Geometry check sheet. Reference: the model listing, model coordinates, mm. A direction names the side the tool comes from. Round coordinates to 2 decimals unless told otherwise and drop trailing zeros. Loops run counter-clockwise (first coordinate to the right, second up) from the corner with the lowest first, then second, coordinate; pieces in that order, holes last. Notation, with made-up numbers: (68.5, 46.25) - (81.5, 46.25) arc R24 cw to (81.5, 77.25) - close; hole circle Ø9 at (-38.75, 20). An arc over 180 degrees is marked (long way). Answer as CSV lines item,"result". Start each with the question number.
1) Cross-section at D-D on y = -22.25. Record the boundary of the cut face in (x, z).
2) Draft check along X on faces 4 (the flat face through (12.565, -13, 19)), 5 (the flat face through (-7, -25.4, 9)), 6 (the cylindrical face through (-44.58, -12.42, 6.44)). Enter one of: released by +X, released by -X, zero draft, split by the parting line, or undercut.
3) Cross-section at A-A on z = 8.5. Record the boundary of the cut face in (x, y).
4) Cross-section at B-B on y = -15.5. Record the boundary of the cut face in (x, z), and give its area (3 significant figures).
5) Cross-section at C-C on z = 28.5. Record the boundary of the cut face in (x, y), and give its area (3 significant figures).
6) Access from +Z, -Z, +X, -X, +Y, -Y to the whole of each face (thin tool, end or side, straight path). Record for faces 1 (the flat face through (17, -13, 12.7)), 2 (the cylindrical face through (20.226, -16.564, 6.439)), 3 (the flat face through (-32, -15, 12.7)).
7) Depth check by flat-ended pin: P1, Ø5, axis at x = -22.5, z = 29.5, coming from the +Y side; P2, Ø10, axis at x = -38.5, y = -5, coming from the +Z side; P3, Ø7.5, axis at x = 25.27, y = -12.7, coming from the -Z side; P4, Ø8, axis at y = -20.5, z = 6.5, coming from the +X side. Enter the tip coordinate at first touch or a pass-through.
8) Thickness scan on line 1 along Y through (x, z) = (-38.5, 10); line 2 along Z through (x, y) = (32.5, -21.5); line 3 along Y through (x, z) = (-33, 11). Record the ranges inside material, lowest first.
from build123d import *

# Parameters (mm, degrees)
F1_DEPTH  = 25.4
F3_DEPTH  = 25.4
F5_DEPTH  = 25.4
F6_R      = 6.35
F7_DEPTH  = 25.4
F8_R      = 6.35
F9_DEPTH  = 25.4
F10_R     = 6.35
F11_DEPTH = 38.1
F13_DEPTH = 38.1


with BuildPart() as f1:
    # F0 (on Front) → F1 (new body)
    with BuildSketch(Plane.XZ):
        Polygon((-50.9347495013, 12.7), (-50.9347495013, 0), (37.9652504987, 0), (37.9652504987, 12.7), (12.5652504987, 12.7), (12.5652504987, 36.2809036063), (-25.5347495013, 36.2809036063), (-25.5347495013, 12.7), align=None)
    extrude(amount=F1_DEPTH)

    # F2 (on face) → F3 (cut)
    with BuildSketch(Plane.XY.offset(12.7)):
        with BuildLine():
            ThreePointArc((-50.9347495013, -12.7), (-47.2150056224, -3.7197438789), (-38.2347495013, 0))
            Line((-38.2347495013, 0), (-50.9347495013, 0))
            Line((-50.9347495013, 0), (-50.9347495013, -12.7))
        make_face()
        with BuildLine():
            Line((-50.9347495013, -25.4), (-38.2347495013, -25.4))
            ThreePointArc((-38.2347495013, -25.4), (-47.2150056224, -21.6802561211), (-50.9347495013, -12.7))
            Line((-50.9347495013, -12.7), (-50.9347495013, -25.4))
        make_face()
    extrude(amount=-F3_DEPTH, mode=Mode.SUBTRACT)

    # F4 (on face) → F5 (cut)
    with BuildSketch(Plane.XY.offset(12.7)):
        with BuildLine():
            ThreePointArc((25.2652504987, 0), (34.2455066198, -3.7197438789), (37.9652504987, -12.7))
            Line((37.9652504987, -12.7), (37.9652504987, 0))
            Line((37.9652504987, 0), (25.2652504987, 0))
        make_face()
        with BuildLine():
            Line((37.9652504987, -25.4), (37.9652504987, -12.7))
            ThreePointArc((37.9652504987, -12.7), (34.2455066198, -21.6802561211), (25.2652504987, -25.4))
            Line((25.2652504987, -25.4), (37.9652504987, -25.4))
        make_face()
    extrude(amount=-F5_DEPTH, mode=Mode.SUBTRACT)

    # F6 (on face) → F7 (cut)
    with BuildSketch(Plane.XY.offset(12.7)):
        with Locations((-38.2347495013, -12.7)):
            Circle(F6_R)
    extrude(amount=-F7_DEPTH, mode=Mode.SUBTRACT)

    # F8 (on face) → F9 (cut)
    with BuildSketch(Plane.XY.offset(12.7)):
        with Locations((25.2652504987, -12.7)):
            Circle(F8_R)
    extrude(amount=-F9_DEPTH, mode=Mode.SUBTRACT)

    # F10 (on face) → F11 (cut)
    with BuildSketch(Plane.YZ.offset(12.5652504987)):
        with Locations((-12.7911586314, 26.1209036063)):
            Circle(F10_R)
    extrude(amount=-F11_DEPTH, mode=Mode.SUBTRACT)

    # F12 (on face) → F13 (cut)
    with BuildSketch(Plane.YZ.offset(12.5652504987)):
        with BuildLine():
            ThreePointArc((-25.4, 23.5809036063), (-21.6802561211, 32.5611597274), (-12.7, 36.2809036063))
            Line((-12.7, 36.2809036063), (-25.4, 36.2809036063))
            Line((-25.4, 36.2809036063), (-25.4, 23.5809036063))
        make_face()
        with BuildLine():
            ThreePointArc((-12.7, 36.2809036063), (-3.7197438789, 32.5611597274), (0, 23.5809036063))
            Line((0, 23.5809036063), (0, 36.2809036063))
            Line((0, 36.2809036063), (-12.7, 36.2809036063))
        make_face()
    extrude(amount=-F13_DEPTH, mode=Mode.SUBTRACT)


solid = f1.part
Answer block:
1,outline,"(-46.61, 0) - (33.64, 0) - (33.64, 12.7) - (12.57, 12.7) - (12.57, 31.95) - (-25.53, 31.95) - (-25.53, 12.7) - (-46.61, 12.7) - close"
2,face 4,"released by +X"
2,face 5,"zero draft"
2,face 6,"undercut"
3,outline,"(-38.23, -25.4) - (25.27, -25.4) arc R12.7 ccw to (25.27, 0) - (-38.23, 0) arc R12.7 ccw to start; hole circle Ø12.7 at (-38.23, -12.7); hole circle Ø12.7 at (25.27, -12.7)"
4,outline,"(-50.62, 0) - (-43.93, 0) - (-43.93, 12.7) - (-50.62, 12.7) - close; (-32.54, 0) - (19.57, 0) - (19.57, 12.7) - (12.57, 12.7) - (12.57, 20.38) - (-25.53, 20.38) - (-25.53, 12.7) - (-32.54, 12.7) - close; (-25.53, 31.86) - (12.57, 31.86) - (12.57, 35.97) - (-25.53, 35.97) - close; (30.96, 0) - (37.65, 0) - (37.65, 12.7) - (30.96, 12.7) - close"
4,area,"1,280 mm^2"
5,outline,"(-25.53, -24.41) - (12.57, -24.41) - (12.57, -18.68) - (-25.53, -18.68) - close; (-25.53, -6.9) - (12.57, -6.9) - (12.57, -0.99) - (-25.53, -0.99) - close"
5,area,"444 mm^2"
6,face 1,"+Z, +X, +Y, -Y"
6,face 2,"+Z, -Z"
6,face 3,"+Z, -X, +Y, -Y"
7,P1,"stops at y = -0.47"
7,P2,"stops at z = 12.7"
7,P3,"passes through"
7,P4,"stops at x = 37.38"
8,line 1,"y = -25.4 to -19.04, -6.36 to 0"
8,line 2,"z = 0 to 12.7"
8,line 3,"y = -25.4 to -16.29, -9.11 to 0"
